Check sheet for the modelled part. Datum: model origin and axes. Units: mm. Coordinates: 2 decimals unless noted, no trailing zeros. Order: outer loops, then holes, each group sorted by start corner. A loop starts at its lowest first (then second) coordinate and runs counter-clockwise, first axis right, second up. Notation, with made-up numbers: (77, 79.25) -> (114, 79.25) arc R7 cw to (114, 87.25) -> close; hole circle Ø5 at (6.25, 56.25). An arc over 180 degrees is marked (long way). Put each result on its own line as item: value. Start each with the question number.
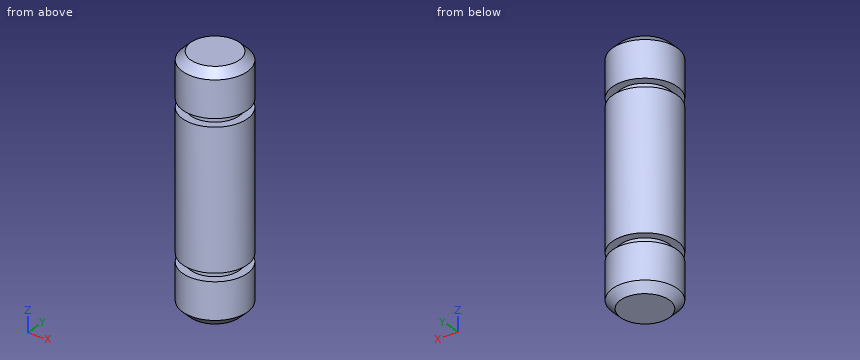
```python
from build123d import *

# Parameters (mm, degrees)
SKETCH_1_R          = 8
EXTRUDE_1_DEPTH     = 60
CHAMFER_1_SIZE      = 2
SKETCH_3_OUTSIDE_W  = 30.824
SKETCH_3_OUTSIDE_H  = 30.824
SKETCH_3_OUTSIDE_R  = 6
CUT_EXTRUDE_1_DEPTH = 2
SKETCH_4_OUTSIDE_W  = 30.824
SKETCH_4_OUTSIDE_H  = 30.824
SKETCH_4_OUTSIDE_R  = 6
CUT_EXTRUDE_2_DEPTH = 2


with BuildPart() as part:
    # 草图1 → 凸台-拉伸1 (new body)
    with BuildSketch(Plane.XY):
        Circle(SKETCH_1_R)
    extrude(amount=EXTRUDE_1_DEPTH)

    # 倒角1
    chamfer_1_edges = [part.edges().sort_by_distance(p)[0] for p in [
        (-8, 0, 0),
        (-8, 0, 60),
    ]]
    chamfer(chamfer_1_edges, length=CHAMFER_1_SIZE)

    # 草图3 outside → 切除-拉伸1 (cut)
    with BuildSketch(Plane.XY.offset(13)):
        Rectangle(SKETCH_3_OUTSIDE_W, SKETCH_3_OUTSIDE_H)
        Circle(SKETCH_3_OUTSIDE_R, mode=Mode.SUBTRACT)
    extrude(amount=-CUT_EXTRUDE_1_DEPTH, mode=Mode.SUBTRACT)

    # 草图4 outside → 切除-拉伸2 (cut)
    with BuildSketch(Plane.XY.offset(47)):
        Rectangle(SKETCH_4_OUTSIDE_W, SKETCH_4_OUTSIDE_H)
        Circle(SKETCH_4_OUTSIDE_R, mode=Mode.SUBTRACT)
    extrude(amount=CUT_EXTRUDE_2_DEPTH, mode=Mode.SUBTRACT)


solid = part.part
```
1) Scan lines: line 1 along Z through (x, y) = (3.75, 5.75); line 2 along Z through (x, y) = (-5.25, -4.25); line 3 along X through (y, z) = (-0.25, 57.5). Record each from-to range of solid material in increasing order. Write a range as [from, to].
2) Sectioned sample at C-C (z = 50). Record the boundary of the cut face in (x, y), plus the area to 3 significant figures.
3) Sectioned sample at A-A (y = 0). Record the boundary of the cut face in (x, z), plus the area to 3 significant figures.
4) Gauge pin test, flat ends, axial feed: pin 1 (2 mm diameter, centred on y = 2.5, z = 10, fed in from -X); pin 2 (3 mm diameter, centred on x = -4.5, z = 38.5, fed in from -Y). Record the tip position at first contact, or that the pin passes through.
Entries:
1. line 1: z = [0.86, 11], [13, 47], [49, 59.14]
1. line 2: z = [0.75, 11], [13, 47], [49, 59.25]
1. line 3: x = [-8, 8]
2. outline: circle Ø16 at (0, 0)
2. area: 201 mm2
3. outline: (-8, 2) -> (-6, 0) -> (6, 0) -> (8, 2) -> (8, 11) -> (6, 11) -> (6, 13) -> (8, 13) -> (8, 47) -> (6, 47) -> (6, 49) -> (8, 49) -> (8, 58) -> (6, 60) -> (-6, 60) -> (-8, 58) -> (-8, 49) -> (-6, 49) -> (-6, 47) -> (-8, 47) -> (-8, 13) -> (-6, 13) -> (-6, 11) -> (-8, 11) -> close
3. area: 936 mm2
4. pin 1: stops at x = -7.86
4. pin 2: stops at y = -7.42
